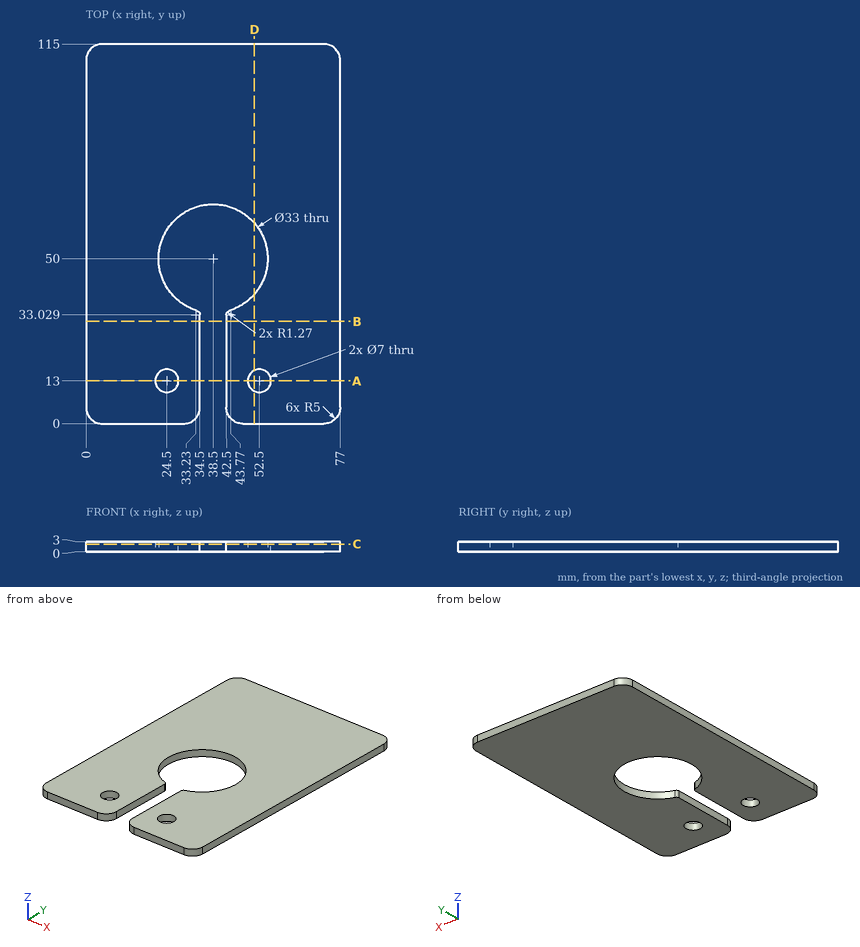
Can you work these out from the drawing? Everything is in mm from the part's minimum corner. Coordinates: 2 decimals unless noted, no trailing zeros. Loops run counter-clockwise (first coordinate to the right, second up) from the corner with the lowest first, then second, coordinate; pieces in that order, holes last.
1) Imagine slicing it at A-A (y = 13). List the corners of the cut face in (x, z) for me, and give its area (3 significant figures).
Reported:
outline: (0, 0) - (21, 0) - (21, 3) - (0, 3) - close; (28, 0) - (34.5, 0) - (34.5, 3) - (28, 3) - close; (42.5, 0) - (49, 0) - (49, 3) - (42.5, 3) - close; (56, 0) - (77, 0) - (77, 3) - (56, 3) - close
area: 165 mm2
2) Imagine slicing it at D-D (x = 51). List the corners of the cut face in (y, z) for me.
Reported:
outline: (0, 0) - (9.84, 0) - (9.84, 3) - (0, 3) - close; (16.16, 0) - (39.23, 0) - (39.23, 3) - (16.16, 3) - close; (60.77, 0) - (115, 0) - (115, 3) - (60.77, 3) - close
3) Imagine slicing it at B-B (y = 31). List the corners of the cut face in (x, z) for me, and give its area (3 significant figures).
Reported:
outline: (0, 0) - (34.5, 0) - (34.5, 3) - (0, 3) - close; (42.5, 0) - (77, 0) - (77, 3) - (42.5, 3) - close
area: 207 mm2
4) Please list where these lines run through material, in increasing order: line 1 along X through (y, z) = (50, 1.25); line 2 along Y through (x, z) = (52.5, 1.65) (1 decimal); line 3 along X through (y, z) = (37.5, 1.5).
Reported:
line 1: x = 0 to 22, 55 to 77
line 2: y = 0 to 9.5, 16.5 to 41.3, 58.7 to 115
line 3: x = 0 to 27.73, 49.27 to 77
5) Imagine slicing it at C-C (z = 2.3). List the corners of the cut face in (x, y) for me, and give its area (3 significant figures).
Reported:
outline: (0, 5) arc R5 ccw to (5, 0) - (29.5, 0) arc R5 ccw to (34.5, 5) - (34.5, 33.03) arc R1.27 ccw to (33.61, 34.24) arc R16.5 cw (long way) to (43.39, 34.24) arc R1.27 ccw to (42.5, 33.03) - (42.5, 5) arc R5 ccw to (47.5, 0) - (72, 0) arc R5 ccw to (77, 5) - (77, 110) arc R5 ccw to (72, 115) - (5, 115) arc R5 ccw to (0, 110) - close; hole circle Ø7 at (24.5, 13); hole circle Ø7 at (52.5, 13)
area: 7,620 mm2
